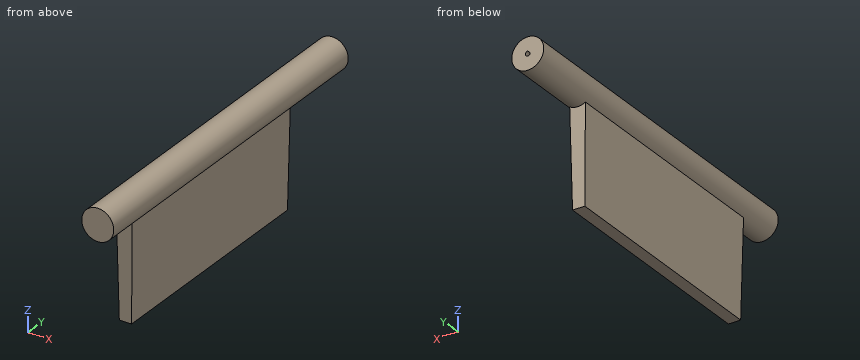
from build123d import *

# Parameters (mm, degrees)
SKIZZE2_R                       = 10
AUFSATZ_LINEAR_AUSTRAGEN1_DEPTH = 210
SKIZZE7_W                       = 10.134043554
SKIZZE7_H                       = 150
AUFSATZ_LINEAR_AUSTRAGEN2_DEPTH = 70
AUFSATZ_LINEAR_AUSTRAGEN2_DRAFT = -1
SKIZZE8_R                       = 10
AUFSATZ_LINEAR_AUSTRAGEN3_DEPTH = 12
SCHNITT_LINEAR_AUSTRAGEN1_DEPTH = 10


with BuildPart() as part:
    # Skizze2 → Aufsatz-Linear austragen1 (new body)
    with BuildSketch(Plane(origin=(0, 0, 0), x_dir=(1, 0, 0), z_dir=(0, 1, 0))):
        with Locations(Location((0, 0, 0), (0, 0, 270))):
            Circle(SKIZZE2_R)
    extrude(amount=AUFSATZ_LINEAR_AUSTRAGEN1_DEPTH)


with BuildPart() as aufsatz_linear_austragen2_tool:
    # Skizze7 → Aufsatz-Linear austragen2 (with draft: the straight prism first)
    with BuildSketch(Plane.XY):
        with Locations((0, 100)):
            Rectangle(SKIZZE7_W, SKIZZE7_H)
    extrude(amount=-AUFSATZ_LINEAR_AUSTRAGEN2_DEPTH)
    # Aufsatz-Linear austragen2: the draft: its side faces are tilted about the plane it starts from
    aufsatz_linear_austragen2_sides = [aufsatz_linear_austragen2_tool.faces().sort_by_distance(p)[0] for p in [
        (0, 175, -35),
        (-5.067021777, 100, -35),
        (0, 25, -35),
        (5.067021777, 100, -35),
    ]]
    draft(aufsatz_linear_austragen2_sides, Plane.XY, AUFSATZ_LINEAR_AUSTRAGEN2_DRAFT)


with BuildPart() as part_1:
    add(part.part)

    # Aufsatz-Linear austragen2: add aufsatz_linear_austragen2_tool
    add(aufsatz_linear_austragen2_tool.part)

    # Skizze8 → Aufsatz-Linear austragen3 (add)
    with BuildSketch(Plane(origin=(0, 210, 0), x_dir=(1, 0, 0), z_dir=(0, 1, 0))):
        with Locations(Location((0, 0, 0), (0, 0, 270))):
            Circle(SKIZZE8_R)
    extrude(amount=AUFSATZ_LINEAR_AUSTRAGEN3_DEPTH)

    # Skizze9 → Schnitt-Linear austragen1 (cut)
    with BuildSketch(Plane(origin=(0, 222, 0), x_dir=(1, 0, 0), z_dir=(0, 1, 0))):
        with BuildLine():
            Line((0, -1.5), (-1.5, 0))
            ThreePointArc((-1.5, 0), (1.060660172, 1.060660172), (0, -1.5))
        make_face()
    extrude(amount=-SCHNITT_LINEAR_AUSTRAGEN1_DEPTH, mode=Mode.SUBTRACT)


solid = part_1.part
Read the model definition and answer for the solid it produces. Units are mm, in the model's axes. Give positions to 0.01 mm unless a question says otherwise; leave off trailing zeros. Write each loop counter-clockwise with the first axis right and the second up, starting at its lowest first coordinate (ties: lowest second). Pieces come first, ordered by that corner, then holes. Notation, with made-up numbers: (-18.5, 39) - (-5.5, 39) arc R31 ccw to (-5.5, 63) - close; hole circle Ø7 at (66.5, 77.5). An arc over 180 degrees is marked (long way). Use CSV: the item, a comma, the result in double quotes. Start each with the question number.
Item 1: Consider line 1 (X direction, y = 219.25, z = 0); line 2 (Y direction, x = -4, z = -10); line 3 (Z direction, x = 0.25, y = 38). Determine where each line is inside the solid, lowest interval first.
Item 2: The part is cut by section B-B, the plane z = -55. Give the vertices of the cut face in (x, y).
Item 3: Flat-ended cylindrical pins translate along their axes: P1, Ø3, axis at x = 4.5, y = 165, coming from the +Z side; P2, Ø2, axis at y = 117.5, z = -43, coming from the +X side; P3, Ø1.5, axis at x = -1.5, y = 192, coming from the -Z side; P4, Ø3, axis at x = -8, z = -14.5, coming from the +Y side. Find the tip coordinate at first contact, or state that the pin passes through.
Item 4: The part is cut by section A-A, the plane y = 54. Give the vertices of the cut face in (x, z) (3 decimals).
Taken from the geometry:
1,line 1,"-10 to -1.5, 1.5 to 10"
1,line 2,"25.17 to 174.83"
1,line 3,"-70 to 10"
2,outline,"(-4.11, 25.96) - (4.11, 25.96) - (4.11, 174.04) - (-4.11, 174.04) - close"
3,P1,"z = 9.54"
3,P2,"x = 4.33"
3,P3,"z = -9.97"
3,P4,"through"
4,outline,"(-4.915, -8.709) - (-3.845, -70) - (3.845, -70) - (4.915, -8.709) arc R10 ccw (long way) to start"
